Check sheet for the modelled part. Datum: model origin and axes. Units: mm. Face numbers are marked on the shaded views. A direction names the side the tool comes from. Give positions to 0.01 mm unless a question says otherwise; leave off trailing zeros. Loops run counter-clockwise (first coordinate to the right, second up) from the corner with the lowest first, then second, coordinate; pieces in that order, holes last.
```python
from build123d import *

# Parameters (mm, degrees)
SKETCH1_R           = 8
SKETCH1_R_2         = 2.54
BOSS_EXTRUDE1_DEPTH = 8
SKETCH2_R           = 8
SKETCH2_R_2         = 5.08
CUT_EXTRUDE1_DEPTH  = 5.4


with BuildPart() as part:
    # Sketch1 → Boss-Extrude1 (new body)
    with BuildSketch(Plane(origin=(0, 0, 0), x_dir=(1, 0, 0), z_dir=(0, 1, 0))):
        with Locations(Location((0, 0, 0), (0, 0, 270))):
            Circle(SKETCH1_R)
        with Locations(Location((0, 0, 0), (0, 0, 270))):
            Circle(SKETCH1_R_2, mode=Mode.SUBTRACT)
    extrude(amount=BOSS_EXTRUDE1_DEPTH)

    # Sketch2 → Cut-Extrude1 (cut)
    with BuildSketch(Plane(origin=(0, 1.3, 0), x_dir=(1, 0, 0), z_dir=(0, 1, 0))):
        with Locations(Location((0, 0, 0), (0, 0, 270))):
            Circle(SKETCH2_R)
        with Locations(Location((0, 0, 0), (0, 0, 90))):
            Circle(SKETCH2_R_2, mode=Mode.SUBTRACT)
    extrude(amount=CUT_EXTRUDE1_DEPTH, mode=Mode.SUBTRACT)


solid = part.part
```
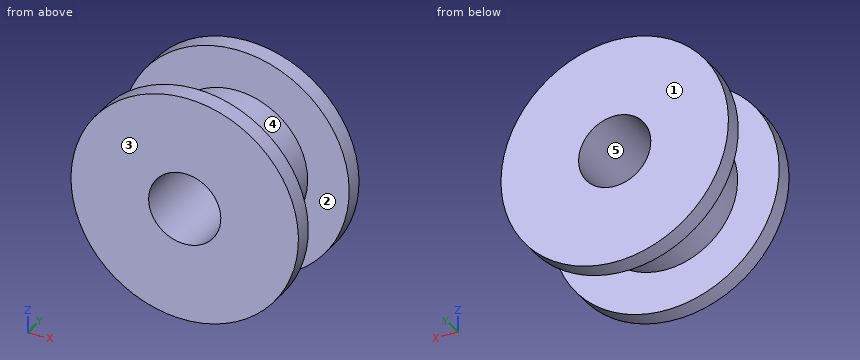
(1) Access from +Z, -Z, +X, -X, +Y, -Y to the whole of each face (thin tool, end or side, straight path). Record for the marked faces 4 and 5.
(2) Section check B-B on z = 0. Record the boundary of the cut face in (x, y), plus the area to 3 significant figures.
(3) Section check D-D on z = -4.5. Record the boundary of the cut face in (x, y).
(4) Release check for a two-part mould opening along Y. For the marked faces 1, 2 and 3 record: pulls with the +Y half, pulls with the -Y half, needs draft (parallel to the pull), parting line crosses it, or undercut.
(5) Section check A-A on x = 0. Record the boundary of the cut face in (y, z).
(6) Section check C-C on y = 7.5. Record the boundary of the cut face in (x, z).
(7) Gauge pin test, flat ends, axial feed: pin 1 Ø2 at (y, z) = (5.5, 0.5) entering from +X; pin 2 Ø3 at (x, z) = (0, 0) entering from -Y; pin 3 Ø1 at (x, y) = (-2.5, 4.5) entering from -Z; pin 4 Ø1 at (y, z) = (4.5, 2.5) entering from -X. Record the tip position at first contact, or that the pin passes through.
(8) Material ranges on line 1 (Y direction, x = -6.5, z = 2); line 2 (X direction, y = 6.75, z = 0); line 3 (X direction, y = 2.75, z = 0), recorded low to high.
Computed values:
1. face 4: none
1. face 5: +Y, -Y
2. outline: (-8, 0) - (-2.54, 0) - (-2.54, 8) - (-8, 8) - (-8, 6.7) - (-5.08, 6.7) - (-5.08, 1.3) - (-8, 1.3) - close; (2.54, 0) - (8, 0) - (8, 1.3) - (5.08, 1.3) - (5.08, 6.7) - (8, 6.7) - (8, 8) - (2.54, 8) - close
2. area: 55.8 mm2
3. outline: (-6.61, 0) - (6.61, 0) - (6.61, 1.3) - (2.36, 1.3) - (2.36, 6.7) - (6.61, 6.7) - (6.61, 8) - (-6.61, 8) - (-6.61, 6.7) - (-2.36, 6.7) - (-2.36, 1.3) - (-6.61, 1.3) - close
4. face 1: pulls with the +Y half
4. face 2: undercut
4. face 3: pulls with the -Y half
5. outline: (0, -8) - (1.3, -8) - (1.3, -5.08) - (6.7, -5.08) - (6.7, -8) - (8, -8) - (8, -2.54) - (0, -2.54) - close; (0, 2.54) - (8, 2.54) - (8, 8) - (6.7, 8) - (6.7, 5.08) - (1.3, 5.08) - (1.3, 8) - (0, 8) - close
6. outline: circle Ø16 at (0, 0); hole circle Ø5.08 at (0, 0)
7. pin 1: stops at x = 5.08
7. pin 2: passes through
7. pin 3: stops at z = -4.67
7. pin 4: stops at x = -4.67
8. line 1: y = 0 to 1.3, 6.7 to 8
8. line 2: x = -8 to -2.54, 2.54 to 8
8. line 3: x = -5.08 to -2.54, 2.54 to 5.08
